Work out the finished part from the listing and answer in its coordinate system (mm). A direction names the side the tool comes from. Round coordinates to 2 decimals unless told otherwise and drop trailing zeros. Write each loop counter-clockwise with the first axis right and the second up, starting at its lowest first coordinate (ties: lowest second). Pieces come first, ordered by that corner, then holes. Notation, with made-up numbers: M 65,15 L 93,15 A26 ccw 93,43 Z; hole C 79.25,49.25 d11. An arc over 180 degrees is marked long. One line per item, written item: value. Start each with the question number.
Q1. Find section B-B (z = -3.75). Write down the section's boundary in (x, y).
Q2. A tool of negligible diameter and unlimited length cuts with its end or side. For faces 3 (the flat face through (11.5, -24, -4)), 4 (the flat face through (-12.3, 0, 0)), 5 (the flat face through (-8.5, 23.8, 3.6)), 6 (the flat face through (11.5, 25, 5)), from which of +Z, -Z, +X, -X, +Y, -Y can it reach the whole face along a straight path? Write none if from no direction.
Q3. Find section C-C (y = -13.5). Write down the section's boundary in (x, z), and give its area (3 significant figures).
Q4. Given pin 1 Ø12 at (x, y) = (-11, -8) entering from -Z; pin 2 Ø3 at (x, y) = (-9.5, 10.5) entering from +Z; pin 3 Ø1.7 at (y, z) = (-21.5, 4.5) entering from -X, each flat-ended and moving along its own axis, determine where each tip first touches the part or whether it passes through.
Q5. Consider probe 1 along Z at (x, y) = (8, -16); probe 2 along X at (y, z) = (0.5, -0.5); probe 3 along Y at (x, z) = (-8.75, -6). Determine where each line is inside the solid, lowest interval first.
Q6. The mould has two halves that part along Y. Classify faces 1 (the flat face through (-10.5, 24, 4.1)), 2 (the flat face through (0, 25, 6.6)): released by +Y, released by -Y, zero draft, split by the parting line, or undercut.
Autodesk Inventor part; units mm, degrees
ref_plane "YZ Plane" through (0, 0, 0) normal (1, 0, 0) x (0, 1, 0)
ref_plane "XZ Plane" through (0, 0, 0) normal (0, 1, 0) x (-1, 0, 0)
ref_plane "XY Plane" through (0, 0, 0) normal (0, 0, 1) x (1, 0, 0)
sketch "Skizze2" plane through (0, 0, 0) normal (0, 1, 0) x (-1, 0, 0)
  line L0 (-12.3, -2.3) -> (12.3, -2.3)
  line L1 (12.3, -2.3) -> (12.3, 2.3)
  line L2 (12.3, 2.3) -> (-12.3, 2.3)
  line L3 (-12.3, 2.3) -> (-12.3, -2.3)
  line L4 (-12.3, -2.3) -> (12.3, 2.3) construction
  line L5 (12.3, -2.3) -> (-12.3, 2.3) construction
  line L6 (-12, 3.1) -> (12, 3.1)
  line L7 (12, -3.1) -> (-12, -3.1)
  line L8 (-19.5039, 0) -> (19.5039, 0)
  line L9 (0, -4.8039) -> (0, 4.8039)
  arc A0 (-12, 3.1) -> (-13.6, 1.5) centre (-12, 1.5) ccw
  arc A1 (-13.6, -1.5) -> (-12, -3.1) centre (-12, -1.5) ccw
  arc A2 (13.6, 1.5) -> (12, 3.1) centre (12, 1.5) ccw
  arc A3 (12, -3.1) -> (13.6, -1.5) centre (12, -1.5) ccw
  line L10 (-13.6, 1.5) -> (-13.6, -1.5)
  line L11 (13.6, 1.5) -> (13.6, -1.5)
  point P0 (0, 0)
  dimension "d0" = 24.6
  dimension "d1" = 4.6
  dimension "d2" = 0.8
  dimension "d29" = 3.2
  dimension "d32" = 1.3
extrude "Extrusion1" add sketch "Skizze2" along normal blind 25.9 contours L0 L9 L7 A1 L10 L8 L3 | L0 L1 L8 L11 A3 L7 L9 | L8 L10 A0 L6 L9 L2 L3 | L1 L2 L9 L6 A2 L11 L8
sketch "Skizze3" plane through (0, 25.9, 0) normal (0, 1, 0) x (1, 0, 0)
  line L0 (12.3, 2.3) -> (12.3, -2.3)
  line L1 (12.3, -2.3) -> (-12.3, -2.3)
  line L2 (-12.3, -2.3) -> (-12.3, 2.3)
  line L3 (-12.3, 2.3) -> (12.3, 2.3)
  line L4 (12, 3.1) -> (-12, 3.1)
  line L5 (-12, -3.1) -> (12, -3.1)
  line L6 (19.0715, 0) -> (-19.0452, 0)
  line L7 (11.5, -3.1) -> (-11.5, -3.1)
  line L8 (-11.5, -3.1) -> (-11.5, -6.6)
  line L9 (-11.5, -6.6) -> (11.5, -6.6)
  line L10 (11.5, -6.6) -> (11.5, -3.1)
  line L11 (12, 3.1) -> (-12, 3.1)
  line L12 (11.5, 3.1) -> (-11.5, 3.1)
  line L13 (-11.5, 3.1) -> (-11.5, 6.6)
  line L14 (-11.5, 6.6) -> (11.5, 6.6)
  line L15 (11.5, 6.6) -> (11.5, 3.1)
  line L16 (0, 7.84) -> (0, -7.84)
  line L17 (-12, -3.1) -> (12, -3.1)
  arc A0 (12, -3.1) -> (13.6, -1.5) centre (12, -1.5) ccw
  arc A1 (13.6, 1.5) -> (12, 3.1) centre (12, 1.5) ccw
  arc A2 (-12, 3.1) -> (-13.6, 1.5) centre (-12, 1.5) ccw
  arc A3 (-13.6, -1.5) -> (-12, -3.1) centre (-12, -1.5) ccw
  line L18 (13.6, -1.5) -> (13.6, 1.5)
  line L19 (-13.6, 1.5) -> (-13.6, -1.5)
  dimension "d18" = 3.5
  dimension "d19" = 23
extrude "Extrusion2" add sketch "Skizze3" against normal blind 2.5 contours L16 L14 L15 L4 | L4 L13 L14 L16 | L16 L9 L8 L5 | L5 L10 L9 L16
mirror "Spiegeln1" about plane through (0, 0, 0) normal (0, 1, 0) of "Extrusion1", "Extrusion2"
chamfer "Fase1" distance 3.5 angle 45 2 edges at (0, -23.4, 3.1) (0, -23.4, -3.1)
sketch "Skizze7" plane through (0, 23.4, 0) normal (0, -1, 0) x (1, 0, 0)
  line L0 (13.4387, -2.2) -> (13.6, -2.2)
  line L1 (13.6, 1.5) -> (13.6, 2.2)
  line L2 (13.6, 2.2) -> (13.4387, 2.2)
  line L3 (11.5, 3.1) -> (11.5, 6.6)
  line L4 (11.5, 6.6) -> (-11.5, 6.6)
  line L5 (-11.5, 6.6) -> (-11.5, 3.1)
  line L6 (11.5, 3.1) -> (-11.5, 3.1)
  line L7 (-11.5, -3.1) -> (11.5, -3.1)
  line L8 (-11.5, -3.1) -> (-11.5, -6.6)
  line L9 (-11.5, -6.6) -> (11.5, -6.6)
  line L10 (11.5, -6.6) -> (11.5, -3.1)
  line L11 (-13.6, -2.2) -> (-13.4387, -2.2)
  line L12 (-13.4387, 2.2) -> (-13.6, 2.2)
  line L13 (-13.6, -1.5) -> (-13.6, -2.2)
  line L14 (-13.6, 2.2) -> (-13.6, 1.5)
  arc A0 (-13.6, -1.5) -> (-13.4387, -2.2) centre (-12, -1.5) ccw
  arc A1 (-13.4387, 2.2) -> (-13.6, 1.5) centre (-12, 1.5) ccw
  arc A2 (13.4387, -2.2) -> (13.6, -1.5) centre (12, -1.5) ccw
  line L15 (13.6, -2.2) -> (13.6, -1.5)
  arc A3 (13.6, 1.5) -> (13.4387, 2.2) centre (12, 1.5) ccw
extrude "Extrusion4" [suppressed]
chamfer "Fase2" [suppressed]
sketch "Skizze8" plane through (-11.5, 23.4, 3.1) normal (0, 0, 1) x (1, 0, 0)
  line L0 (0, 2.5) -> (23, 2.5)
  line L1 (0, 2.5) -> (0, 0)
  line L2 (23, 0) -> (0, 0)
  line L3 (23, 2.5) -> (23, 0)
  line L4 (0, 0) -> (23, 0)
  line L5 (0, 0) -> (0, 1)
  line L6 (0, 1) -> (5, 0)
  line L7 (5, 0) -> (0, 0)
  point P0 (11.5, -23.4)
  dimension "d33" = 1
  dimension "d34" = 5
extrude "Extrusion5" cut sketch "Skizze8" along normal blind 1 contours L6 L2 L1
sketch "Skizze9" plane through (-11.5, 25.9, 3.1) normal (-1, 0, 0) x (0, 0, 1)
  line L0 (0, -1.5) -> (1, -1.5)
  line L1 (1, -1.5) -> (1, -2.5)
  line L2 (3.5, -2.5) -> (1, -2.5)
  line L3 (3.5, 0) -> (3.5, -2.5)
  line L4 (0, 0) -> (3.5, 0)
  line L5 (0, -1.5) -> (0, 0)
  line L6 (1, -2.5) -> (0, -2.5)
  line L7 (0, -2.5) -> (0, 0)
  line L8 (0, 0) -> (1, 0)
  line L9 (1, 0) -> (1, -2.5)
  point P0 (-3.1, -25.9)
extrude "Extrusion6" cut sketch "Skizze9" against normal blind 1 contours L5 L4 L9 L0 | L0 L1 L6 L7
chamfer "Fase3" distance 0.2 angle 45 16 edges at (0, 25.9, 6.6) (11.5, 25.9, 4.85) (13.1314, 25.9, 2.6314) (13.6, 25.9, 0) (13.1314, 25.9, -2.6314) (11.75, 25.9, -3.1) (11.75, 25.9, 3.1) (11.5, 25.9, -4.85) (0, 25.9, -6.6) (-11.5, 25.9, -4.85) (-11.75, 25.9, -3.1) (-13.1314, 25.9, -2.6314) (-13.6, 25.9, 0) (-13.1314, 25.9, 2.6314) (-11.25, 25.9, 3.1) (-11.5, 25.9, 5.35)
properties part number "Spulenkoerper" material "PC/ABS-Kunststoff"
The answers:
1. outline: M -11.5,-25.9 L 11.5,-25.9 L 11.5,-20.55 L -11.5,-20.55 Z; M -11.5,23.4 L 11.5,23.4 L 11.5,25.7 L 11.3,25.9 L -11.3,25.9 L -11.5,25.7 Z
2. face 3: -Z, +X, +Y, -Y
2. face 4: +Y, -Y
2. face 5: -X
2. face 6: +Z, +X, +Y, -Y
3. outline: M -13.6,-1.5 A1.6 ccw -12,-3.1 L 12,-3.1 A1.6 ccw 13.6,-1.5 L 13.6,1.5 A1.6 ccw 12,3.1 L -12,3.1 A1.6 ccw -13.6,1.5 Z; hole M -12.3,-2.3 L 12.3,-2.3 L 12.3,2.3 L -12.3,2.3 Z
3. area: 53.3 mm2
4. pin 1: z = -3.1
4. pin 2: z = 3.1
4. pin 3: x = -11.5
5. probe 1: -3.1 to -2.3, 2.3 to 3.1
5. probe 2: -13.6 to -12.3, 12.3 to 13.6
5. probe 3: -25.9 to -22.8, 23.4 to 25.9
6. face 1: undercut
6. face 2: zero draft
